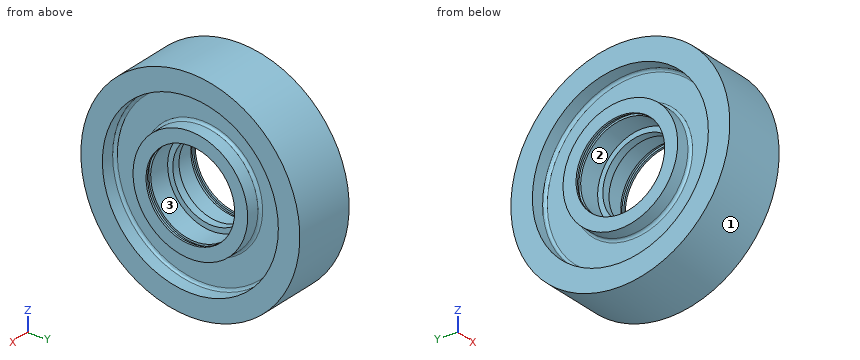
```python
from build123d import *


with BuildPart() as f1:
    # F0 (on Front) → F1 (revolve)
    with BuildSketch(Plane.XZ):
        with BuildLine():
            Line((0, 76.2), (0, 213.36))
            Line((0, 213.36), (-60.96, 213.36))
            Line((-60.96, 213.36), (-60.96, 171.45))
            Line((-60.96, 171.45), (-35.56, 171.45))
            ThreePointArc((-35.56, 171.45), (-31.967898, 169.962102), (-30.48, 166.37))
            Line((-30.48, 166.37), (-30.48, 116.84))
            ThreePointArc((-30.48, 116.84), (-31.967898, 113.247898), (-35.56, 111.76))
            Line((-35.56, 111.76), (-60.96, 111.76))
            Line((-60.96, 111.76), (-60.96, 86.36))
            Line((-60.96, 86.36), (-57.15, 86.36))
            Line((-57.15, 86.36), (-57.15, 90.17))
            Line((-57.15, 90.17), (-49.53, 90.17))
            Line((-49.53, 90.17), (-49.53, 86.36))
            Line((-49.53, 86.36), (-7.62, 86.36))
            Line((-7.62, 86.36), (-7.62, 76.2))
            Line((-7.62, 76.2), (0, 76.2))
        make_face()
        with BuildLine():
            Line((60.96, 213.36), (0, 213.36))
            Line((0, 213.36), (0, 76.2))
            Line((0, 76.2), (7.62, 76.2))
            Line((7.62, 76.2), (7.62, 86.36))
            Line((7.62, 86.36), (49.53, 86.36))
            Line((49.53, 86.36), (49.53, 90.17))
            Line((49.53, 90.17), (57.15, 90.17))
            Line((57.15, 90.17), (57.15, 86.36))
            Line((57.15, 86.36), (60.96, 86.36))
            Line((60.96, 86.36), (60.96, 111.76))
            Line((60.96, 111.76), (35.56, 111.76))
            ThreePointArc((35.56, 111.76), (31.967898, 113.247898), (30.48, 116.84))
            Line((30.48, 116.84), (30.48, 166.37))
            ThreePointArc((30.48, 166.37), (31.967898, 169.962102), (35.56, 171.45))
            Line((35.56, 171.45), (60.96, 171.45))
            Line((60.96, 171.45), (60.96, 213.36))
        make_face()
    revolve(axis=Axis((-30.48, 0, 0), (-1, 0, 0)))


solid = f1.part
```
Check sheet for the modelled part. Datum: model origin and axes. Units: mm. Face numbers are marked on the shaded views. A direction names the side the tool comes from. Round coordinates to 2 decimals unless told otherwise and drop trailing zeros. Loops run counter-clockwise (first coordinate to the right, second up) from the corner with the lowest first, then second, coordinate; pieces in that order, holes last. Notation, with made-up numbers: (66, 21.5) -> (71, 21.5) arc R13 cw to (71, 34.5) -> close; hole circle Ø2 at (87.25, -22.5). An arc over 180 degrees is marked (long way). Write item = value, one per line. Start each with the question number.
1) Thickness scan on probe 1 along Z at (x, y) = (52, -3); probe 2 along Y at (x, z) = (-15, 0); probe 3 along Y at (x, z) = (42.5, 0). Record the ranges inside material, lowest first.
2) Set-up check for the marked faces 1, 2 and 3: record each of +Z, -Z, +X, -X, +Y, -Y from which the full face is reachable in a straight line by a thin tool's end or side.
3) Gauge pin test, flat ends, axial feed: pin 1 Ø12 at (x, y) = (18.5, -156.5) entering from +Z; pin 2 Ø4 at (y, z) = (-45.5, -105.5) entering from +X; pin 3 Ø5 at (x, y) = (15.5, 149) entering from +Z. Record the tip position at first contact, or that the pin passes through.
4) Sectioned sample at B-B, the plane x = -16. Record the cut outline in (y, z), plus the area to 3 significant figures.
5) Sectioned sample at A-A, the plane x = 43.5. Record the cut outline in (y, z), plus the area to 3 significant figures.
Results are:
q1.probe_1 = -213.34 to -171.42, -111.72 to -90.12, 90.12 to 111.72, 171.42 to 213.34
q1.probe_2 = -213.36 to -86.36, 86.36 to 213.36
q1.probe_3 = -213.36 to -171.45, -111.76 to -86.36, 86.36 to 111.76, 171.45 to 213.36
q2.face_1 = +X, -X
q2.face_2 = -X
q2.face_3 = +X
q3.pin_1 = 151.24
q3.pin_2 = 32.36
q3.pin_3 = 155.11
q4.outline = circle Ø426.72 at (0, 0); hole circle Ø172.72 at (0, 0)
q4.area = 120,000 mm^2
q5.outline = circle Ø426.72 at (0, 0); circle Ø223.52 at (0, 0); hole circle Ø342.9 at (0, 0); hole circle Ø172.72 at (0, 0)
q5.area = 66,500 mm^2
